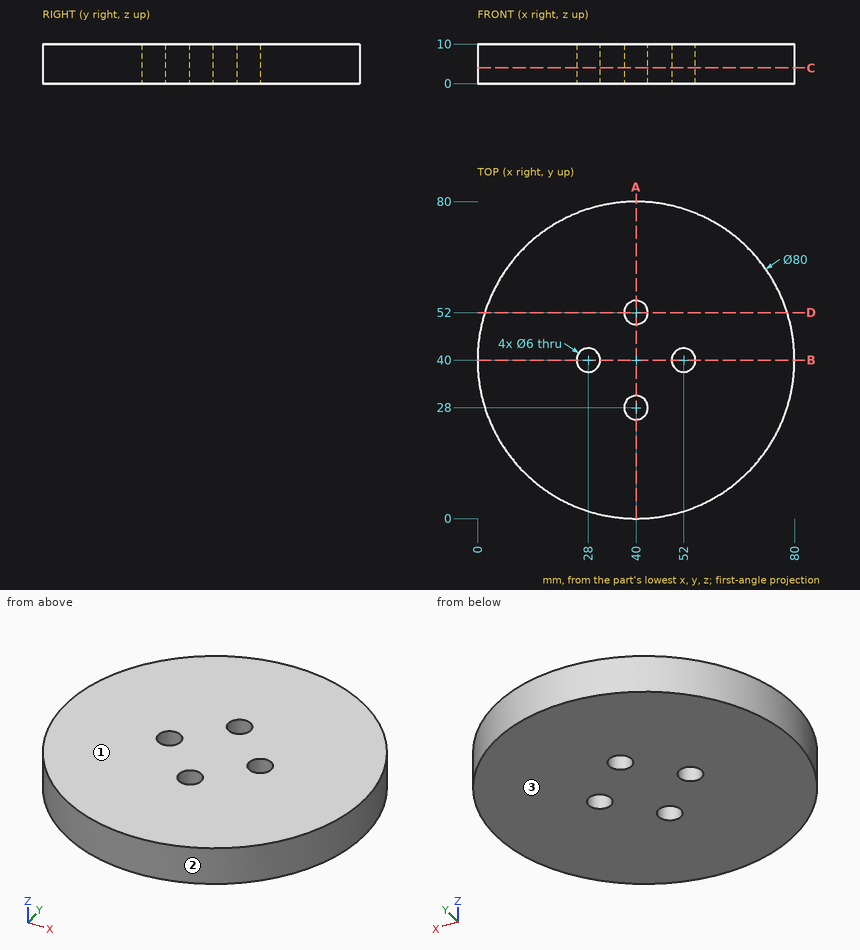
Can you work these out from the drawing? Everything is in mm from the part's minimum corner. Give positions to 0.01 mm unless a question says otherwise; leave off trailing zeros. Order: outer loops, then holes, each group sorted by start corner. A loop starts at its lowest first (then second) coordinate and runs counter-clockwise, first axis right, second up. Notation, with made-up numbers: (38.5, 5) -> (47.5, 5) arc R25 ccw to (47.5, 28) -> close; hole circle Ø11 at (-37, -22). An arc over 180 degrees is marked (long way). Return JSON: item names as keys, results as strings.
1. Imagine slicing it at D-D on y = 52. List the corners of the cut face in (x, z) for me.
Answer list:
{"outline": "(1.84, 0) -> (37, 0) -> (37, 10) -> (1.84, 10) -> close; (43, 0) -> (78.16, 0) -> (78.16, 10) -> (43, 10) -> close"}
2. I need wall thicknesses on line 1 (Y direction, x = 40, z = 3.25); line 2 (X direction, y = 52.5, z = 9.5); line 3 (X direction, y = 41.5, z = 1.75). Which ranges of each line are inside material? Lowest first, please. Write a range as from..to.
Answer list:
{"line 1": "y = 0..25, 31..49, 55..80", "line 2": "x = 2..37.04, 42.96..78", "line 3": "x = 0.03..25.4, 30.6..49.4, 54.6..79.97"}
3. Imagine slicing it at A-A on x = 40. List the corners of the cut face in (y, z) for me, then the cut area to 3 significant figures.
Answer list:
{"outline": "(0, 0) -> (25, 0) -> (25, 10) -> (0, 10) -> close; (31, 0) -> (49, 0) -> (49, 10) -> (31, 10) -> close; (55, 0) -> (80, 0) -> (80, 10) -> (55, 10) -> close", "area": "680 mm2"}
4. Imagine slicing it at C-C on z = 4. List the corners of the cut face in (x, y) for me, then the cut area to 3 significant figures.
Answer list:
{"outline": "circle Ø80 at (40, 40); hole circle Ø6 at (28, 40); hole circle Ø6 at (40, 28); hole circle Ø6 at (40, 52); hole circle Ø6 at (52, 40)", "area": "4,910 mm2"}
5. For pin 1 Ø6 at (y, z) = (18, 6) entering from -X; pin 2 Ø1 at (y, z) = (9.5, 4) entering from +X; pin 3 Ø5.5 at (x, y) = (40, 28) entering from +Z; pin 4 Ø1 at (y, z) = (49, 4.5) entering from +X, each with a flat end and sliding along its axis, tell me the tip position at first contact or that it passes through.
Answer list:
{"pin 1": "stops at x = 4.8", "pin 2": "stops at x = 66.46", "pin 3": "passes through", "pin 4": "stops at x = 79.09"}
6. Thinking about a two-plate mould opening in Z: for the marked faces 1, 2 and 3, which applies, pulls with the +Z half, pulls with the -Z half, needs draft (parallel to the pull), parting line crosses it, or undercut?
Answer list:
{"face 1": "pulls with the +Z half", "face 2": "needs draft", "face 3": "pulls with the -Z half"}
